Can you work these out from the model? Positions are in its coordinate system, mm. A direction names the side the tool comes from. Give positions to 0.01 mm unless a question says otherwise; leave off trailing zeros. Order: outer loops, then holes, each group sorted by start corner. A loop starts at its lowest first (then second) coordinate and runs counter-clockwise, first axis right, second up.
Item 1: Which directions (+Z, -Z, +X, -X, +Y, -Y) give clear straight access to the entire face, cutting with the end or side of a thin tool? Please do faces 4 (the flat face through (76, -2.54, 0)), 5 (the cylindrical face through (146.52, -1.25, -0.49)).
Item 2: I want a section at B-B, the plane x = 18.5. Write out the boundary of the cut face in (y, z).
Item 3: I'm going to push flat-ended pins straight in: pin 1 Ø0.8 at (x, z) = (141.5, -0.5) entering from -Y; pin 2 Ø1.5 at (x, y) = (36.5, -2) entering from -Z. Where does each tip first touch, or does it pass through?
Item 4: If we mould it in two halves opening along X, with no side actions, what happens to faces 1 (the flat face through (42, -0.254, 0)), 2 (the flat face through (46, -2.54, 0)), 3 (the cylindrical face through (75.564, -1.381, 0.858))? For each: +X half, -X half, draft (parallel to the pull), parting line (faces both ways), or undercut.
Item 5: If I drill on line 1 along Y through (x, z) = (75, -0.85); line 2 along Z through (x, y) = (6.5, -1.15); line 3 along Z through (x, y) = (131, -2.25), over which ranges is the centre line in solid material (lowest first)?
Item 6: I want a section at A-A, the plane y = -1.65. Count the separate pieces of the cut face and the enclosed holes in it, then the cut area to 3 significant figures.
```python
from build123d import *

# Parameters (mm, degrees)
F0_R     = 1.27
F1_DEPTH = 2.54
F3_DEPTH = 0.254


with BuildPart() as f1:
    # F0 (on Front) → F1 (new body)
    with BuildSketch(Plane.XZ):
        Circle(F0_R)
        with Locations((7.649997, 0)):
            Circle(F0_R)
        with Locations((15.299995, 0)):
            Circle(F0_R)
        with Locations((22.949992, 0)):
            Circle(F0_R)
        with Locations((30.59999, 0)):
            Circle(F0_R)
        with Locations((38.249987, 0)):
            Circle(F0_R)
        with Locations((45.899984, 0)):
            Circle(F0_R)
        with Locations((53.549982, 0)):
            Circle(F0_R)
        with Locations((61.199979, 0)):
            Circle(F0_R)
        with Locations((68.849977, 0)):
            Circle(F0_R)
        with Locations((76.499974, 0)):
            Circle(F0_R)
        with Locations((84.149971, 0)):
            Circle(F0_R)
        with Locations((91.799969, 0)):
            Circle(F0_R)
        with Locations((99.449966, 0)):
            Circle(F0_R)
        with Locations((107.099964, 0)):
            Circle(F0_R)
        with Locations((114.749961, 0)):
            Circle(F0_R)
        with Locations((122.399958, 0)):
            Circle(F0_R)
        with Locations((130.049956, 0)):
            Circle(F0_R)
        with Locations((137.699953, 0)):
            Circle(F0_R)
        with Locations((145.349951, 0)):
            Circle(F0_R)
    extrude(amount=F1_DEPTH)

    # F2 (on Front) → F3 (join)
    with BuildSketch(Plane.XZ):
        Polygon((0, -1.27), (145.349951, -1.27), (145.349951, 0), (145.349951, 1.27), (0, 1.27), align=None)
    extrude(amount=F3_DEPTH)


solid = f1.part
```
Results list:
1. face 4: +Z, -Z, +X, -X, -Y
1. face 5: -Y
2. outline: (-0.25, -1.27) - (0, -1.27) - (0, 1.27) - (-0.25, 1.27) - close
3. pin 1: stops at y = -0.25
3. pin 2: stops at z = -0.78
4. face 1: undercut
4. face 2: draft
4. face 3: undercut
5. line 1: y = -0.25 to 0
5. line 2: z = -0.54 to 0.54
5. line 3: z = -0.84 to 0.84
6. separate pieces: 20
6. enclosed holes: 0
6. area: 101 mm2
